Study the drawing (mm; zero at the part's minimum x, y, z) and answer. A direction names the side the tool comes from. Round coordinates to 2 decimals unless told otherwise and drop trailing zeros. Order: outer loops, then holes, each group sorted by start corner. A loop starts at its lowest first (then second) coordinate and runs counter-clockwise, first axis right, second up. Notation, with made-up numbers: (76.25, 38) - (121.25, 38) arc R29 ccw to (121.25, 75) - close; hole circle Ø7 at (-9.5, 19). An arc over 180 degrees is marked (long way). Put each result on its own line as item: value. Start each with the question number.
Q1. Find the intervals of material crossed by line 1 along Y through (x, z) = (16.8, 12.5); line 2 along Y through (x, z) = (8, 5); line 3 along X through (y, z) = (15, 3), in increasing order. Write a range as from..to.
Q2. Each of these flat-tipped pins is pushed along its axis until it touches: pin 1 Ø4.5 at (x, z) = (8, 8.5) entering from +Y; pin 2 Ø1.5 at (y, z) = (18, 20.5) entering from -X. Where does it stop, or does it pass through?
Q3. For a pull along X with two mould halves and no side action, classify the marked faces 4, 5 and 6 as pulls with the +X half, pulls with the -X half, needs draft (parallel to the pull), parting line crosses it, or undercut.
Q4. Section C-C on x = 8 is taken. Give the vertices of the cut face in (y, z).
Q5. Section D-D on z = 1.5 is taken. Give the vertices of the cut face in (x, y).
Q6. Section A-A on y = 28 is taken. Give the vertices of the cut face in (x, z), then the cut area to 3 significant figures.
Q7. Section B-B on z = 12.5 is taken. Give the vertices of the cut face in (x, y).
Q8. Which of the six approach directions +Z, -Z, +X, -X, +Y, -Y give full straight-line access (tool end or side, diameter ignored) to the marked faces 1, 2 and 3?
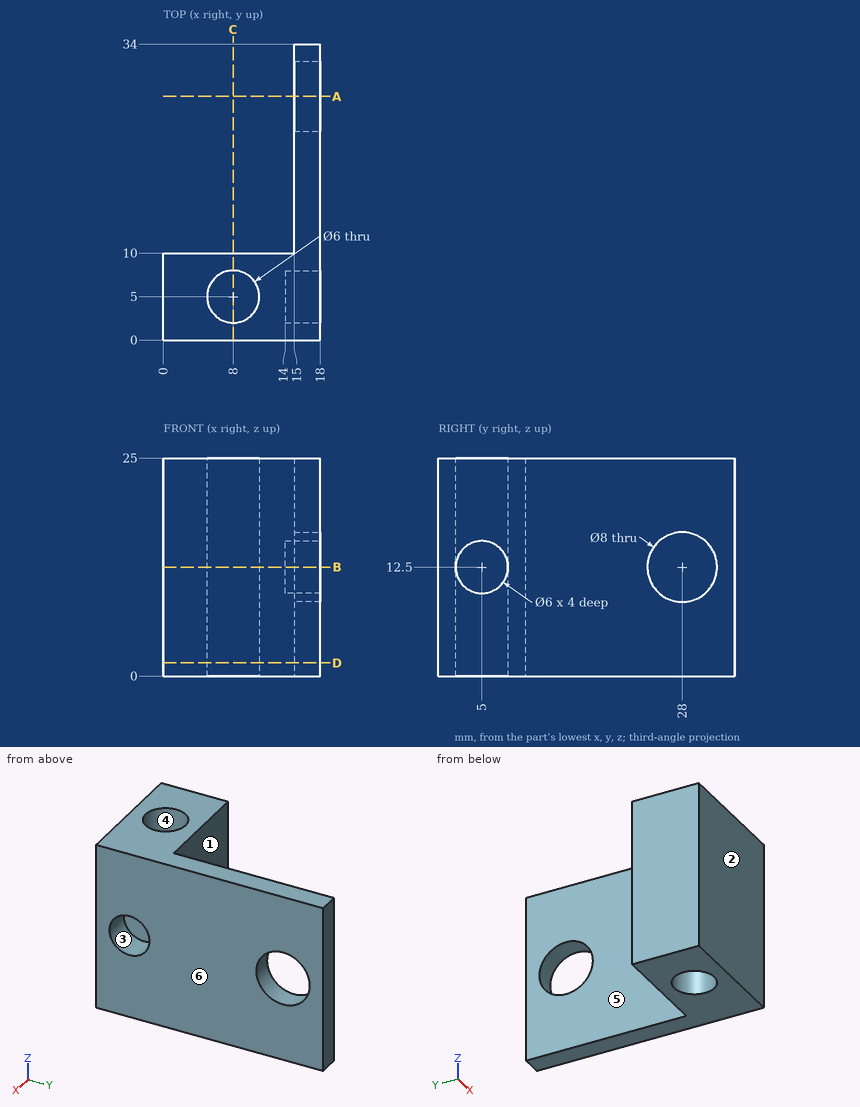
Findings:
1. line 1: 0..2, 8..24, 32..34
1. line 2: 0..2, 8..10
1. line 3: 15..18
2. pin 1: y = 10
2. pin 2: x = 15
3. face 4: undercut
3. face 5: pulls with the -X half
3. face 6: pulls with the +X half
4. outline: (0, 0) - (2, 0) - (2, 25) - (0, 25) - close; (8, 0) - (10, 0) - (10, 25) - (8, 25) - close
5. outline: (0, 0) - (18, 0) - (18, 34) - (15, 34) - (15, 10) - (0, 10) - close; hole circle Ø6 at (8, 5)
6. outline: (15, 0) - (18, 0) - (18, 8.5) - (15, 8.5) - close; (15, 16.5) - (18, 16.5) - (18, 25) - (15, 25) - close
6. area: 51.0 mm2
7. outline: (0, 0) - (18, 0) - (18, 2) - (14, 2) - (14, 8) - (18, 8) - (18, 24) - (15, 24) - (15, 10) - (0, 10) - close; (15, 32) - (18, 32) - (18, 34) - (15, 34) - close; hole circle Ø6 at (8, 5)
8. face 1: +Z, -Z, -X, +Y
8. face 2: +Z, -Z, +X, -X, -Y
8. face 3: +X
